from build123d import *

# Parameters (mm, degrees)
SKETCH_1_R      = 2.5
EXTRUDE_1_DEPTH = 2


with BuildPart() as part:
    # 草图1 → 凸台-拉伸1 (new body)
    with BuildSketch(Plane.XY):
        with BuildLine():
            Line((-35, 4), (-39.799497484, 4))
            ThreePointArc((-39.799497484, 4), (-34.641016151, 20), (-23.363850357, 32.467375879))
            Line((-23.363850357, 32.467375879), (-20.964101615, 28.310889132))
            ThreePointArc((-20.964101615, 28.310889132), (-15.5, 26.846787517), (-14.035898385, 32.310889132))
            Line((-14.035898385, 32.310889132), (-16.435647127, 36.467375879))
            ThreePointArc((-16.435647127, 36.467375879), (0, 40), (16.435647127, 36.467375879))
            Line((16.435647127, 36.467375879), (14.035898385, 32.310889132))
            ThreePointArc((14.035898385, 32.310889132), (15.5, 26.846787517), (20.964101615, 28.310889132))
            Line((20.964101615, 28.310889132), (23.363850357, 32.467375879))
            ThreePointArc((23.363850357, 32.467375879), (34.641016151, 20), (39.799497484, 4))
            Line((39.799497484, 4), (35, 4))
            ThreePointArc((35, 4), (31, 0), (35, -4))
            Line((35, -4), (39.799497484, -4))
            ThreePointArc((39.799497484, -4), (34.641016151, -20), (23.363850357, -32.467375879))
            Line((23.363850357, -32.467375879), (20.964101615, -28.310889132))
            ThreePointArc((20.964101615, -28.310889132), (15.5, -26.846787517), (14.035898385, -32.310889132))
            Line((14.035898385, -32.310889132), (16.435647127, -36.467375879))
            ThreePointArc((16.435647127, -36.467375879), (0, -40), (-16.435647127, -36.467375879))
            Line((-16.435647127, -36.467375879), (-14.035898385, -32.310889132))
            ThreePointArc((-14.035898385, -32.310889132), (-15.5, -26.846787517), (-20.964101615, -28.310889132))
            Line((-20.964101615, -28.310889132), (-23.363850357, -32.467375879))
            ThreePointArc((-23.363850357, -32.467375879), (-34.641016151, -20), (-39.799497484, -4))
            Line((-39.799497484, -4), (-35, -4))
            ThreePointArc((-35, -4), (-31, 0), (-35, 4))
        make_face()
        Circle(SKETCH_1_R, mode=Mode.SUBTRACT)
    extrude(amount=EXTRUDE_1_DEPTH)


solid = part.part
Check sheet for the modelled part. Datum: model origin and axes. Units: mm. A direction names the side the tool comes from. Round coordinates to 2 decimals unless told otherwise and drop trailing zeros. Write each loop counter-clockwise with the first axis right and the second up, starting at its lowest first coordinate (ties: lowest second). Pieces come first, ordered by that corner, then holes. Notation, with made-up numbers: (5.5, -3.75) -> (49.5, -3.75) arc R18 ccw to (49.5, 14.25) -> close; hole circle Ø8 at (55.5, -5). An arc over 180 degrees is marked (long way). Answer as CSV lines item,"result". Start each with the question number.
1) Go/stop test with flat-tipped pins: P1, Ø1, axis at x = -24.5, z = 1.5, coming from the -Y side; P2, Ø1, axis at x = 10, z = 1.5, coming from the +Y side; P3, Ø1, axis at x = 11, z = 1.5, coming from the +Y side. Record where each tip stops, or that it passes through.
2) Material ranges on line 1 (Y direction, x = 0, z = 0.8); line 2 (Y direction, x = 16, z = 0.2); line 3 (X direction, y = 30, z = 0.75), recorded low to high. Write a range as from..to.
3) Section check B-B on y = 0. Enter the section's corners in (x, z), and give its area (3 significant figures).
4) Section check A-A on x = 0. Enter the section's corners in (y, z), and give its area (3 significant figures).
5) Section check D-D on y = -10. Enter the section's corners in (x, z).
6) Release check for a two-part mould opening along X. For faces 4 (the cylindrical face through (-31, 0, 1)), 5 (the cylindrical face through (-15.424, -26.892, 0.986)), 6 (the flat face through (37, -4, 1)) record: pulls with the +X half, pulls with the -X half, needs draft (parallel to the pull), parting line crosses it, or undercut.
7) Section check C-C on z = 1.1. Enter the section's corners in (x, y), and give its area (3 significant figures).
8) Tool access check on faces 1 (the cylindrical face through (-15.58, 26.8, 0.99)), 2 (the flat face through (22.18, -30.42, 0.99)), 3 (the flat face through (-22.18, 30.42, 0.99)). Record the directions out of +Z, -Z, +X, -X, +Y, -Y that give a thin tool (end or side, any length) a straight path to the whole face; none if there is none.
Found:
1,P1,"stops at y = -32"
1,P2,"stops at y = 38.86"
1,P3,"stops at y = 38.6"
2,line 1,"y = -40..-2.5, 2.5..40"
2,line 2,"y = -36.66..-35.71, -26.6..26.6, 35.71..36.66"
2,line 3,"x = -26.46..-21.94, -13.51..13.51, 21.94..26.46"
3,outline,"(-31, 0) -> (-2.5, 0) -> (-2.5, 2) -> (-31, 2) -> close; (2.5, 0) -> (31, 0) -> (31, 2) -> (2.5, 2) -> close"
3,area,"114 mm^2"
4,outline,"(-40, 0) -> (-2.5, 0) -> (-2.5, 2) -> (-40, 2) -> close; (2.5, 0) -> (40, 0) -> (40, 2) -> (2.5, 2) -> close"
4,area,"150 mm^2"
5,outline,"(-38.73, 0) -> (38.73, 0) -> (38.73, 2) -> (-38.73, 2) -> close"
6,face 4,"pulls with the -X half"
6,face 5,"undercut"
6,face 6,"needs draft"
7,outline,"(-39.8, -4) arc R40 ccw to (-23.36, -32.47) -> (-20.96, -28.31) arc R4 cw to (-14.04, -32.31) -> (-16.44, -36.47) arc R40 ccw to (16.44, -36.47) -> (14.04, -32.31) arc R4 cw to (20.96, -28.31) -> (23.36, -32.47) arc R40 ccw to (39.8, -4) -> (35, -4) arc R4 cw to (35, 4) -> (39.8, 4) arc R40 ccw to (23.36, 32.47) -> (20.96, 28.31) arc R4 cw to (14.04, 32.31) -> (16.44, 36.47) arc R40 ccw to (-16.44, 36.47) -> (-14.04, 32.31) arc R4 cw to (-20.96, 28.31) -> (-23.36, 32.47) arc R40 ccw to (-39.8, 4) -> (-35, 4) arc R4 cw to (-35, -4) -> close; hole circle Ø5 at (0, 0)"
7,area,"4,620 mm^2"
8,face 1,"+Z, -Z"
8,face 2,"+Z, -Z, -Y"
8,face 3,"+Z, -Z, +Y"
